For this review, take the finished solid that the model builds, in its own axes (mm). Round coordinates to 2 decimals unless told otherwise and drop trailing zeros. Write each loop counter-clockwise with the first axis right and the second up, starting at its lowest first coordinate (ties: lowest second). Pieces come first, ordered by that corner, then holes. Notation, with made-up numbers: (38.25, -22) - (66.25, -22) arc R33 cw to (66.25, 11) - close; hole circle Ø10 at (-12.5, 3.25). An arc over 180 degrees is marked (long way). One line per item, written item: value. Start each with the question number.
Q1. Add section A-A on z = -0.5. Write out the cut boundary in (x, y), and give its area (3 significant figures).
Q2. Add section B-B on x = 0.5. Write out the cut boundary in (y, z), and give its area (3 significant figures).
Q3. Clearance check with a flat-ended pin moving along its axis: pin 1 Ø2.5 at (x, z) = (0.5, -99.5) entering from +Y. State where the tip first meets the part, or that it passes through.
Q4. For probe 1 along X at (y, z) = (1.5, -7.46); probe 2 along X at (y, z) = (2.25, -99.5); probe 3 along Z at (x, y) = (0.5, 0.9), list the stretches that pass through material, from the lowest coordinate up.
Autodesk Fusion 360 part; units mm, degrees
sketch "Sketch1" plane through (0, 0, 0) normal (0, 1, 0) x (1, 0, 0)
  circle A0 centre (0.5, 99.5) radius 1.6662
  circle A1 centre (7.805, 92.54) radius 1.375
  circle A2 centre (42.195, 92.54) radius 1.375
  circle A3 centre (49.5, 99.5) radius 1.6662
  circle A4 centre (7.805, 7.46) radius 1.375
  circle A5 centre (0.5, 0.5) radius 1.6662
  circle A6 centre (42.195, 7.46) radius 1.375
  circle A7 centre (49.5, 0.5) radius 1.6662
  line L0 (-5, -5) -> (55, -5)
  line L1 (55, -5) -> (55, 105)
  line L2 (55, 105) -> (-5, 105)
  line L3 (-5, 105) -> (-5, -5)
  dimension "d5" = 3.3325
  dimension "d8" = 2.75
extrude "Extrude1" add sketch "Sketch1" along normal blind 2.794
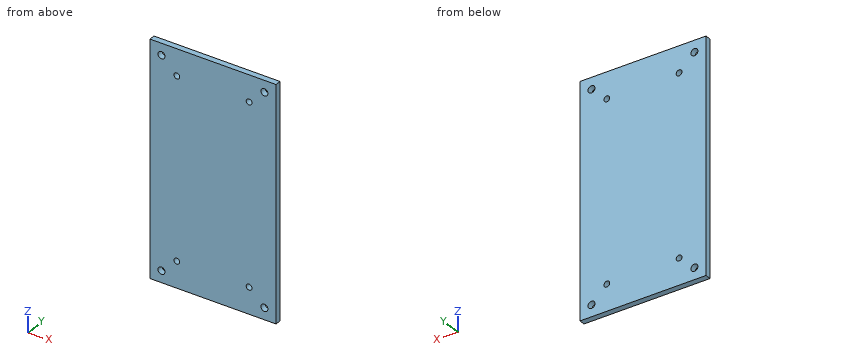
Result set:
1. outline: (-5, 0) - (-1.17, 0) - (-1.17, 2.79) - (-5, 2.79) - close; (2.17, 0) - (47.83, 0) - (47.83, 2.79) - (2.17, 2.79) - close; (51.17, 0) - (55, 0) - (55, 2.79) - (51.17, 2.79) - close
1. area: 149 mm^2
2. outline: (0, -105) - (2.79, -105) - (2.79, -101.17) - (0, -101.17) - close; (0, -97.83) - (2.79, -97.83) - (2.79, -2.17) - (0, -2.17) - close; (0, 1.17) - (2.79, 1.17) - (2.79, 5) - (0, 5) - close
2. area: 289 mm^2
3. pin 1: passes through
4. probe 1: x = -5 to 6.43, 9.18 to 40.82, 43.57 to 55
4. probe 2: x = -5 to -1.17, 2.17 to 47.83, 51.17 to 55
4. probe 3: z = -105 to -101.17, -97.83 to -2.17, 1.17 to 5
